Autodesk Inventor part; units mm, degrees
ref_plane "YZ Plane" through (0, 0, 0) normal (1, 0, 0) x (0, 1, 0)
ref_plane "XZ Plane" through (0, 0, 0) normal (0, 1, 0) x (-1, 0, 0)
ref_plane "XY Plane" through (0, 0, 0) normal (0, 0, 1) x (1, 0, 0)
sketch "Sketch1" plane through (0, 0, 0) normal (0, 1, 0) x (-1, 0, 0)
  line L0 (-36.5, 40) -> (36.5, 40)
  line L1 (36.5, 40) -> (36.5, -40)
  line L2 (36.5, -40) -> (-36.5, -40)
  line L3 (-36.5, -40) -> (-36.5, 40)
  line L4 (-36.5, 40) -> (36.5, -40) construction
  line L5 (36.5, 40) -> (-36.5, -40) construction
  line L6 (36.5, 40) -> (36.5, 13)
  line L7 (-36.5, -40) -> (-9.5, -40)
  line L8 (-36.5, -40) -> (18.5, -40)
  circle A0 centre (8.5, -31.5) radius 1.5
  circle A1 centre (-19.5, -31.5) radius 1.5
  circle A2 centre (-19.5, -31.5) radius 1.5
  circle A3 centre (24, 19) radius 1.5
  line L9 (0, 0) -> (0, 17.5)
  line L10 (0, 17.5) -> (0, 19)
  line L11 (0, 19) -> (24, 19)
  line L12 (0, 0) -> (0, -31.5)
  line L13 (0, -31.5) -> (8.5, -31.5)
  line L14 (0, -31.5) -> (-19.5, -31.5)
  dimension "d0" = 73
  dimension "d1" = 80
  dimension "d5" = 3
  dimension "d6" = 3
  dimension "d7" = 3
  dimension "d10" = 17.5
  dimension "d11" = 8.5
  dimension "d12" = 19.5
  dimension "d13" = 31.5
  dimension "d14" = 24
extrude "Extrusion1" add sketch "Sketch1" along normal blind 8
sketch "Sketch2" plane through (36.5, 0, 40) normal (1, 0, 0) x (0, 0, -1)
  line L0 (75, 0) -> (55, 0)
  line L1 (80, 0) -> (0, 0)
  line L2 (55, 0) -> (35, 0)
  line L3 (0, 0) -> (32.9289, 0)
  line L4 (44.0711, 0) -> (32.9289, 0)
  line L5 (75, 0) -> (80, 0)
  line L6 (5, 0) -> (25, 0)
  line L7 (23.7574, -20) -> (3, -20)
  line L8 (0, -17) -> (0, 0)
  line L9 (0, 0) -> (80, 0)
  line L10 (22.1005, -17) -> (6, -17)
  line L11 (3, -14) -> (3, -2)
  line L12 (3, -2.5) -> (3, -2)
  line L13 (25, 0) -> (45, 0)
  line L14 (25.8787, -19.1213) -> (43.5355, -1.4645)
  line L15 (24.9289, -15.8284) -> (37.3431, -3.4142)
  arc A0 (22.1005, -17) -> (24.9289, -15.8284) centre (22.1005, -13) ccw
  arc A1 (3, -14) -> (6, -17) centre (6, -14) ccw
  arc A2 (0, -17) -> (3, -20) centre (3, -17) ccw
  arc A3 (23.7574, -20) -> (25.8787, -19.1213) centre (23.7574, -17) ccw
  arc A4 (37.3431, -3.4142) -> (35.9289, 0) centre (35.9289, -2) ccw
  arc A5 (5, 0) -> (3, -2) centre (5, -2) ccw
  line L16 (80, 0) -> (47.0711, 0)
  arc A6 (47.0711, 0) -> (43.5355, -1.4645) centre (47.0711, -5) ccw
  line L17 (35.9289, 0) -> (47.0711, 0)
  line L18 (5, 0) -> (0, 0)
  point P0 (40, 0)
  point P1 (39.2426, 0)
  point P2 (25, -20)
  point P3 (0, -20)
  point P4 (40.7574, 0)
extrude "Extrusion3" add sketch "Sketch2" against normal up to surface (73 mm away) contours A6 L14 A3 L7 A2 L8 L1 A5 L11 A1 L10 A0 L15 A4
sketch "Sketch3" plane through (-36.5, 8, 40) normal (0, 0, 1) x (1, 0, 0)
  line L0 (0, 0) -> (28, 0)
  line L1 (0, 0) -> (73, 0)
  line L2 (73, 0) -> (45, 0)
  line L3 (73, -28) -> (0, -28)
  line L4 (28, 0) -> (45, 0)
  line L5 (45, 0) -> (45, -28)
  line L6 (45, -28) -> (28, -28)
  line L7 (28, -28) -> (28, 0)
  line L8 (73, -8) -> (0, -8)
  line L9 (28, 0) -> (45, 0)
  line L10 (45, 0) -> (45, -8)
  line L11 (45, -8) -> (28, -8)
  line L12 (28, -8) -> (28, 0)
  point P0 (36.5, -8)
  dimension "d32" = 28
  dimension "d33" = 28
extrude "Extrusion4" cut sketch "Sketch3" against normal up to surface (80 mm away) contours L8 L5 L3 L7
properties part number "Base"
For this review, take the finished solid that the model builds, in its own axes (mm). A direction names the side the tool comes from. Round coordinates to 2 decimals unless told otherwise and drop trailing zeros. Write each loop counter-clockwise with the first axis right and the second up, starting at its lowest first coordinate (ties: lowest second). Pieces come first, ordered by that corner, then holes. Notation, with made-up numbers: (-4.5, 52.25) - (23.5, 52.25) arc R17 ccw to (23.5, 73.25) - close; hole circle Ø7 at (33, -5). An arc over 180 degrees is marked (long way). Use a Markdown table: item, result.
Q1. We need section B-B (z = -31.5). Give the boundary of the cut face in (x, y), plus the area to 3 significant figures.
Derived:
| item | result |
|---|---|
| outline | (-36.5, 0) - (-10, 0) - (-10, 8) - (-36.5, 8) - close; (-7, 0) - (18, 0) - (18, 8) - (-7, 8) - close; (21, 0) - (36.5, 0) - (36.5, 8) - (21, 8) - close |
| area | 536 mm2 |
Q2. Machinability: for faces 4 (the cylindrical face through (-22.3, -1.27, 2.21)), 5 (the cylindrical face through (-22.89, 3.94, 17.99)), 6 (the flat face through (-22, -10, 5)), 7 (the flat face through (-8.5, -17.5, 23.5)), which of the approach directions +Z, -Z, +X, -X, +Y, -Y give a long, thin tool a straight path to every point of the face, cutting with its end or side? Answer none if there is none.
Derived:
| item | result |
|---|---|
| face 4 | +X, -X |
| face 5 | +Y |
| face 6 | -Z, +X, -X, -Y |
| face 7 | +Z, -Z, -Y |
Q3. We need section A-A (x = 19.5). Give the boundary of the cut face in (y, z).
Derived:
| item | result |
|---|---|
| outline | (-20, 16.24) arc R3 ccw to (-19.12, 14.12) - (-1.46, -3.54) arc R5 cw to (0, -7.07) - (0, -30) - (8, -30) - (8, 40) - (-17, 40) arc R3 ccw to (-20, 37) - close; (0, -40) - (8, -40) - (8, -33) - (0, -33) - close; hole (-17, 17.9) arc R4 ccw to (-15.83, 15.07) - (-3.41, 2.66) arc R2 ccw to (0, 4.07) - (0, 35) arc R2 ccw to (-2, 37) - (-14, 37) arc R3 ccw to (-17, 34) - close |
Q4. Clearance check with flat-ended pins moving along their axes: pin 1 (4 mm diameter, centred on x = -21, y = -14.5, fed in from -Z); pin 2 (3.5 mm diameter, centred on x = -20, y = -6.5, fed in from -Z); pin 3 (10 mm diameter, centred on x = 6, z = -10.5, fed in from -Y); pin 4 (6 mm diameter, centred on y = -13, z = 14.5, fed in from +X). State where each tip first meets the part, or that it passes through.
Derived:
| item | result |
|---|---|
| pin 1 | stops at z = 7.5 |
| pin 2 | stops at z = -0.25 |
| pin 3 | stops at y = -0.08 |
| pin 4 | stops at x = 36.5 |
Q5. Wall thickness on line 1 along Z through (x, y) = (-8.5, 5.5); line 2 along Y through (x, z) = (25, -34.5); line 3 along Z through (x, y) = (-24, 4): over which ranges is each line inside the solid? List them lowest first.
Derived:
| item | result |
|---|---|
| line 1 | z = -40 to -33, -30 to 40 |
| line 2 | y = 0 to 8 |
| line 3 | z = -40 to 17.5, 20.5 to 40 |
Q6. We need section C-C (y = -6). Give the boundary of the cut face in (x, z), plus the area to 3 significant figures.
Derived:
| item | result |
|---|---|
| outline | (-36.5, 1) - (-8.5, 1) - (-8.5, 5.24) - (-36.5, 5.24) - close; (-36.5, 37) - (-8.5, 37) - (-8.5, 40) - (-36.5, 40) - close; (8.5, 1) - (36.5, 1) - (36.5, 5.24) - (8.5, 5.24) - close; (8.5, 37) - (36.5, 37) - (36.5, 40) - (8.5, 40) - close |
| area | 406 mm2 |
Q7. We need section D-D (x = -28). Give the boundary of the cut face in (y, z).
Derived:
| item | result |
|---|---|
| outline | (-20, 16.24) arc R3 ccw to (-19.12, 14.12) - (-1.46, -3.54) arc R5 cw to (0, -7.07) - (0, -40) - (8, -40) - (8, 40) - (-17, 40) arc R3 ccw to (-20, 37) - close; hole (-17, 17.9) arc R4 ccw to (-15.83, 15.07) - (-3.41, 2.66) arc R2 ccw to (0, 4.07) - (0, 35) arc R2 ccw to (-2, 37) - (-14, 37) arc R3 ccw to (-17, 34) - close |
Q8. The part is to be moulded in two halves that separate along Z. For faces 1 (the flat face through (-22, -17, 26)), 2 (the flat face through (8.5, -17.4, 21.8)), 3 (the cylindrical face through (22.7, -0.37, -5.18)), say which applies: pulls with the +Z half, pulls with the -Z half, needs draft (parallel to the pull), parting line crosses it, or undercut.
Derived:
| item | result |
|---|---|
| face 1 | undercut |
| face 2 | needs draft |
| face 3 | pulls with the -Z half |
